```python
from build123d import *

# Parameters (mm, degrees)
SKETCH1_W           = 55
SKETCH1_H           = 33
BOSS_EXTRUDE1_DEPTH = 48
CUT_EXTRUDE1_DEPTH  = 51.5


with BuildPart() as part:
    # Sketch1 → Boss-Extrude1 (new body)
    with BuildSketch(Plane(origin=(0, 0, 0), x_dir=(1, 0, 0), z_dir=(0, 1, 0))):
        Rectangle(SKETCH1_W, SKETCH1_H)
    extrude(amount=BOSS_EXTRUDE1_DEPTH)

    # Sketch2 → Cut-Extrude1 (cut)
    with BuildSketch(Plane.ZY.offset(25.75)):
        with BuildLine():
            Line((14.75565, 32), (14.75565, 16))
            ThreePointArc((14.75565, 16), (0, 1.24435), (-14.75565, 16))
            Line((-14.75565, 16), (-14.75565, 32))
            ThreePointArc((-14.75565, 32), (0, 46.75565), (14.75565, 32))
        make_face()
    extrude(amount=-CUT_EXTRUDE1_DEPTH, mode=Mode.SUBTRACT)


solid = part.part
```
Geometry: final body of the model. Coordinates: model frame, mm. A direction names the side the tool comes from. Coordinates: 2 decimals unless noted, no trailing zeros. Order: outer loops, then holes, each group sorted by start corner. A loop starts at its lowest first (then second) coordinate and runs counter-clockwise, first axis right, second up. Notation, with made-up numbers: (61.5, -6.5) - (65.5, -6.5) arc R21 ccw to (65.5, 0.5) - close; hole circle Ø1 at (0.25, 41). An arc over 180 degrees is marked (long way). Write each question's results on one line, items separated by ' | '.
(1) Set-up query: faces 1 (the face through (-0.361, 46.752, -0.324)), 2 (the face through (27.5, 24, 0)). Return all of +Z, -Z, +X, -X, +Y, -Y with unobstructed straight access to the full face (end or side cutting, diameter ignored); none if empty.
Values found:
face 1: none | face 2: +Z, -Z, +X, +Y, -Y
(2) First-contact query: pin 1 Ø1.5 at (x, z) = (-15.5, -1.5) entering from -Y. Flat tip, straight axial feed; report the tip coordinate or a pass-through.
Values found:
pin 1: stops at y = 0
(3) Section query A-A, the plane x = 23. Return the cut outline in (y, z).
Values found:
outline: (0, -16.5) - (48, -16.5) - (48, 16.5) - (0, 16.5) - close; hole (16, -14.76) - (32, -14.76) arc R14.76 ccw to (32, 14.76) - (16, 14.76) arc R14.76 ccw to start
(4) Mould query, pull axis Z, two halves, no side actions, for faces 3 (the face through (0, 24, -14.756)), 4 (the face through (0, 24, -16.5)), 5 (the face through (-27.5, 24, 0)). Classes: +Z half, -Z half, draft (parallel to the pull), parting line (faces both ways), or undercut.
Values found:
face 3: undercut | face 4: -Z half | face 5: draft
(5) Section query B-B, the plane y = 24. Return the cut outline in (x, z).
Values found:
outline: (-27.5, -16.5) - (27.5, -16.5) - (27.5, 16.5) - (-27.5, 16.5) - close; hole (-25.75, -14.76) - (25.75, -14.76) - (25.75, 14.76) - (-25.75, 14.76) - close
(6) Line query: line 1 (X direction, y = 32, z = -2); line 2 (Z direction, x = -6, y = 21.5); line 3 (Y direction, x = 2, z = 0.5). Output: solid intervals per line, ascending. Write a range as [from, to].
Values found:
line 1: x = [-27.5, -25.75], [25.75, 27.5] | line 2: z = [-16.5, -14.76], [14.76, 16.5] | line 3: y = [0, 1.25], [46.75, 48]
